Can you work these out from the model? Positions are in its coordinate system, mm. Round coordinates to 2 decimals unless told otherwise and drop trailing zeros. Write each loop counter-clockwise with the first axis right and the second up, starting at its lowest first coordinate (ties: lowest second). Pieces come first, ordered by that corner, then holes. Notation, with made-up numbers: (4, 15) -> (16, 15) arc R15 cw to (16, 20) -> close; hole circle Ø6 at (36, 7.25). An arc over 180 degrees is marked (long way). Use CSV: the item, a comma, the result in double quotes.
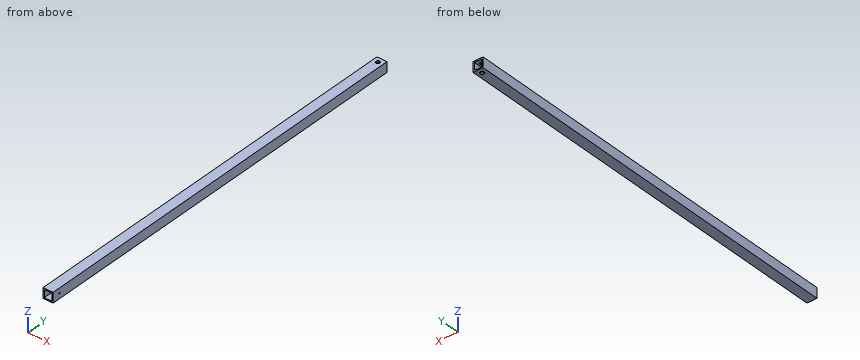
```python
from build123d import *

# Parameters (mm, degrees)
SKETCH1_W               = 12.7
SKETCH1_H               = 12.7
SKETCH1_W_2             = 9.525
SKETCH1_H_2             = 9.525
EXTRUDE_THIN1_DEPTH     = 508
SKETCH3_R               = 2.4765
CUT_EXTRUDE2_DEPTH      = 1
CUT_EXTRUDE2_DEPTH_BACK = 13.7
CUT_EXTRUDE3_REACH      = 14.7
SKETCH4_R               = 0.889


with BuildPart() as part:
    # Sketch1 → Extrude-Thin1 (new body)
    with BuildSketch(Plane(origin=(0, 0, 0), x_dir=(1, 0, 0), z_dir=(0, 1, 0))):
        Rectangle(SKETCH1_W, SKETCH1_H)
        Rectangle(SKETCH1_W_2, SKETCH1_H_2, mode=Mode.SUBTRACT)
    extrude(amount=EXTRUDE_THIN1_DEPTH)

    # Sketch3 → Cut-Extrude2 (cut, two sides)
    with BuildSketch(Plane.XY.offset(6.35)) as cut_extrude2_sk:
        with Locations((0, 501.65)):
            Circle(SKETCH3_R)
    extrude(amount=CUT_EXTRUDE2_DEPTH, mode=Mode.SUBTRACT)
    extrude(cut_extrude2_sk.sketch, amount=-CUT_EXTRUDE2_DEPTH_BACK, mode=Mode.SUBTRACT)

    # Sketch4 → Cut-Extrude3 (cut, up to next)
    with BuildSketch(Plane(origin=(6.35, 0, 0), x_dir=(0, 0, -1), z_dir=(1, 0, 0)), mode=Mode.PRIVATE) as cut_extrude3_sk1:
        with Locations((0, 9.525)):
            Circle(SKETCH4_R)
    cut_extrude3_tool1 = extrude(cut_extrude3_sk1.sketch, amount=-CUT_EXTRUDE3_REACH, mode=Mode.PRIVATE) & part.part
    add(cut_extrude3_tool1.solids().sort_by_distance((6.35, 9.525, 0))[0], mode=Mode.SUBTRACT)


solid = part.part
```
Q1. Will this pin go through, and if not, where does the flat tip stop? P1, Ø3, axis at x = 0, y = 501.65, coming from the -Z side.
Resolved:
P1,"passes through"
Q2. Suppose I cut it at A-A (x = 0). Write out the boundary of the cut face in (y, z).
Resolved:
outline,"(0, -6.35) -> (499.17, -6.35) -> (499.17, -4.76) -> (0, -4.76) -> close; (0, 4.76) -> (499.17, 4.76) -> (499.17, 6.35) -> (0, 6.35) -> close; (504.13, -6.35) -> (508, -6.35) -> (508, -4.76) -> (504.13, -4.76) -> close; (504.13, 4.76) -> (508, 4.76) -> (508, 6.35) -> (504.13, 6.35) -> close"
Q3. Please list where these lines run through material, in increasing order: probe 1 along X at (y, z) = (68, -0.75); probe 2 along X at (y, z) = (501.65, 5.9).
Resolved:
probe 1,"x = -6.35 to -4.76, 4.76 to 6.35"
probe 2,"x = -6.35 to -2.48, 2.48 to 6.35"
Q4. Suppose I cut it at B-B (y = 218.5). Write out the boundary of the cut face in (x, z), and give its area (3 significant figures).
Resolved:
outline,"(-6.35, -6.35) -> (6.35, -6.35) -> (6.35, 6.35) -> (-6.35, 6.35) -> close; hole (-4.76, -4.76) -> (4.76, -4.76) -> (4.76, 4.76) -> (-4.76, 4.76) -> close"
area,"70.6 mm^2"
